Read the model definition and answer for the solid it produces. Units are mm, in the model's axes. Face numbers are marked on the shaded views. A direction names the side the tool comes from. Coordinates: 2 decimals unless noted, no trailing zeros. Loops run counter-clockwise (first coordinate to the right, second up) from the corner with the lowest first, then second, coordinate; pieces in that order, holes last.
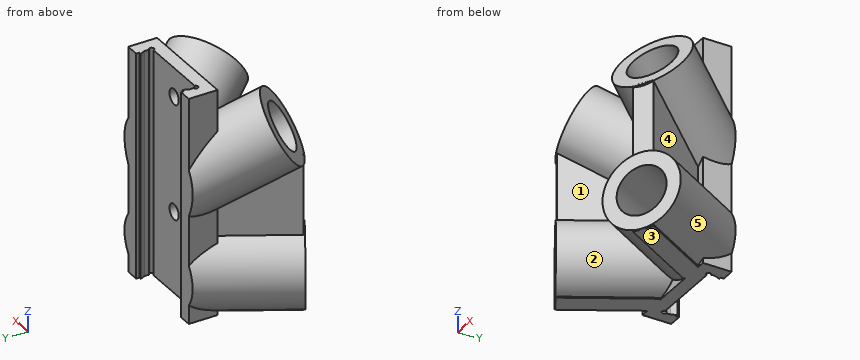
from build123d import *

# Parameters (mm, degrees)
BOSS_EXTRUDE1_DEPTH      = 25
BOSS_EXTRUDE1_DEPTH_BACK = 22
SKETCH5_R                = 8
BOSS_EXTRUDE2_DEPTH      = 30
SKETCH6_R                = 8
BOSS_EXTRUDE3_DEPTH      = 30
SKETCH18_R               = 8
BOSS_EXTRUDE4_DEPTH      = 30
SKETCH19_R               = 8
BOSS_EXTRUDE5_DEPTH      = 30
SKETCH11_R               = 0.5
CUT_EXTRUDE4_DEPTH       = 61.172763276
CUT_EXTRUDE5_REACH       = 41.594
SKETCH12_R               = 1.6
TOPCUT_DEPTH             = 61.172763276
GRABTABS_DEPTH           = 47
BOSS_EXTRUDE6_DEPTH      = 30.5
SKETCH22_R               = 5.1
CUT_EXTRUDE6_DEPTH       = 14
SKETCH23_R               = 5.1
CUT_EXTRUDE7_DEPTH       = 14
SKETCH20_R               = 5.1
CUT_EXTRUDE8_DEPTH       = 14
SKETCH21_R               = 5.1
CUT_EXTRUDE9_DEPTH       = 14


with BuildPart() as part:
    # Sketch3 → Boss-Extrude1 (new, two sides: drawn at the far end of the back side and taken through both)
    with BuildSketch(Plane(origin=(0, 0, 0), x_dir=(-0.9678879191476432, 0.2513821313618881, 0), z_dir=(0, 0, 1)).offset(-BOSS_EXTRUDE1_DEPTH_BACK)):
        Polygon((-7.234103595, -12.967950693), (12.967950693, -7.234103595), (7.234103595, 12.967950693), (-12.967950693, 7.234103595), align=None)
    extrude(amount=BOSS_EXTRUDE1_DEPTH + BOSS_EXTRUDE1_DEPTH_BACK)

    # Sketch5 → Boss-Extrude2 (add)
    with BuildSketch(Plane(origin=(0, 0, 0), x_dir=(-0.7398893525523432, -0.6222846190478576, -0.2555887299474237), z_dir=(0.4497352826512201, -0.740093355961685, 0.499999999999998))):
        with Locations(Location((0, 0, 0), (0, 0, 224.122685504))):
            Circle(SKETCH5_R)
    extrude(amount=BOSS_EXTRUDE2_DEPTH)

    # Sketch6 → Boss-Extrude3 (add)
    with BuildSketch(Plane(origin=(0, 0, 0), x_dir=(-0.7035639492311271, 0.6172392366079582, 0.3521554970945721), z_dir=(-0.4160720061092844, -0.7595288577349761, 0.499999999999998))):
        with Locations(Location((0, 0, 0), (0, 0, 322.705646398))):
            Circle(SKETCH6_R)
    extrude(amount=BOSS_EXTRUDE3_DEPTH)

    # Sketch18 → Boss-Extrude4 (add)
    with BuildSketch(Plane(origin=(0, 0, -14), x_dir=(-0.8770283809411537, 0.48043856945892555, 0), z_dir=(-0.4804385694589255, -0.8770283809411535, 0))):
        with Locations(Location((0, 0, 0), (0, 0, 61.287925102))):
            Circle(SKETCH18_R)
    extrude(amount=BOSS_EXTRUDE4_DEPTH)

    # Sketch19 → Boss-Extrude5 (add)
    with BuildSketch(Plane(origin=(0, 0, -14), x_dir=(-0.8545861965798597, -0.5193095730055144, 0), z_dir=(0.5193095730055143, -0.8545861965798596, 0))):
        with Locations(Location((0, 0, 0), (0, 0, 48.985500334))):
            Circle(SKETCH19_R)
    extrude(amount=BOSS_EXTRUDE5_DEPTH)

    # Sketch11 → Cut-Extrude4 (cut, through all)
    with BuildSketch(Plane(origin=(0, 0, 25), x_dir=(0.967887919147643, -0.25138213136188803, 0), z_dir=(0, 0, 1))):
        with BuildLine():
            ThreePointArc((-4.766381934, -9.44058657), (-4.766628372, -9.424890171), (-4.767367442, -9.409209245))
            Line((-4.767367442, -9.409209245), (-5.339457415, -9.571582654))
            Line((-5.339457415, -9.571582654), (-5.501830825, -8.999492681))
            ThreePointArc((-5.501830825, -8.999492681), (-5.523554594, -9.869378155), (-4.766381934, -9.44058657))
        make_face()
        with BuildLine():
            Line((-5.339457415, -9.571582654), (-4.767367442, -9.409209245))
            ThreePointArc((-4.767367442, -9.409209245), (-5.022796995, -9.003932957), (-5.501830825, -8.999492681))
            Line((-5.501830825, -8.999492681), (-5.339457415, -9.571582654))
        make_face()
        with BuildLine():
            Line((8.999492681, -5.501830825), (9.571582654, -5.339457415))
            Line((9.571582654, -5.339457415), (9.409209245, -4.767367442))
            ThreePointArc((9.409209245, -4.767367442), (9.003932957, -5.022796995), (8.999492681, -5.501830825))
        make_face()
        with BuildLine():
            Line((9.409209245, -4.767367442), (9.571582654, -5.339457415))
            Line((9.571582654, -5.339457415), (8.999492681, -5.501830825))
            ThreePointArc((8.999492681, -5.501830825), (9.561939475, -5.751431903), (9.94058657, -5.266381934))
            ThreePointArc((9.94058657, -5.266381934), (9.782866673, -4.901903771), (9.409209245, -4.767367442))
        make_face()
        with Locations((-5.266381934, -9.44058657)):
            Circle(SKETCH11_R)
        with Locations((9.44058657, -5.266381934)):
            Circle(SKETCH11_R)
        Polygon((-5.339457415, -9.571582654), (9.571582654, -5.339457415), (5.339457415, 9.571582654), (-9.571582654, 5.339457415), align=None)
    extrude(amount=-CUT_EXTRUDE4_DEPTH, mode=Mode.SUBTRACT)

    # Sketch12 → Cut-Extrude5 (cut, up to next)
    with BuildSketch(Plane(origin=(0.235642936, -10.497355496, 0), x_dir=(0.07428415697149086, 0.0016675187230335104, -0.9972357210832067), z_dir=(-0.02244218436129408, 0.9997481424644377, 0)), mode=Mode.PRIVATE) as cut_extrude5_sk1:
        with Locations(Location((-18.947478701, -1.411754543, 0), (0, 0, 274.261167974))):
            Circle(SKETCH12_R)
    cut_extrude5_tool1 = extrude(cut_extrude5_sk1.sketch, amount=CUT_EXTRUDE5_REACH, mode=Mode.PRIVATE) & part.part
    # Sketch12 → Cut-Extrude5 (cut, up to next)
    with BuildSketch(Plane(origin=(0.235642936, -10.497355496, 0), x_dir=(0.07428415697149086, 0.0016675187230335104, -0.9972357210832067), z_dir=(-0.02244218436129408, 0.9997481424644377, 0)), mode=Mode.PRIVATE) as cut_extrude5_sk2:
        with Locations(Location((5.019164388, 0.373972086, 0), (0, 0, 274.261167974))):
            Circle(SKETCH12_R)
    cut_extrude5_tool2 = extrude(cut_extrude5_sk2.sketch, amount=CUT_EXTRUDE5_REACH, mode=Mode.PRIVATE) & part.part
    add(cut_extrude5_tool1.solids().sort_by_distance((0.235643, -10.497355, 19))[0], mode=Mode.SUBTRACT)
    add(cut_extrude5_tool2.solids().sort_by_distance((0.235643, -10.497355, -5.033077))[0], mode=Mode.SUBTRACT)

    # Sketch14 → TopCut (cut, through all)
    with BuildSketch(Plane.XY.offset(25)):
        Polygon((-31.105779731, -5.199391149), (38.352697692, -3.640198499), (37.988721129, 12.574127466), (-33.745248602, 10.963854933), align=None)
    extrude(amount=-TOPCUT_DEPTH, mode=Mode.SUBTRACT)

    # Sketch17 → GrabTabs (add, through all)
    with BuildSketch(Plane(origin=(0, 0, 25), x_dir=(-1, 0, 0), z_dir=(0, 0, -1))):
        Polygon((7.132596783, -5.31140877), (7.607527123, -6.433816222), (7.632470855, -5.322629862), align=None)
        Polygon((-7.888569085, -6.085962364), (-7.363751282, -4.985997097), (-7.863625354, -4.974776005), align=None)
    extrude(amount=GRABTABS_DEPTH)

    # Sketch24 → Boss-Extrude6 (add)
    with BuildSketch(Plane(origin=(0, 0, -22), x_dir=(-1, 0, 0), z_dir=(0, 0, -1))):
        Polygon((-13.818067506, -26.398167405), (-17.409683037, -24.238344439), (-7.909513608, -8.440310713), (-4.317898077, -10.60013368), align=None)
        Polygon((3.837888164, -10.783213448), (7.522803724, -8.786732873), (16.304497418, -24.9951549), (12.619581859, -26.991635476), align=None)
    extrude(amount=-BOSS_EXTRUDE6_DEPTH)

    # Sketch22 → Cut-Extrude6 (cut)
    with BuildSketch(Plane(origin=(-14.413157084, -26.310851428, 0), x_dir=(0.8770283809411535, -0.48043856945892577, 0), z_dir=(-0.4804385694589257, -0.8770283809411534, 0))):
        with Locations((0, -14)):
            Circle(SKETCH22_R)
    extrude(amount=-CUT_EXTRUDE6_DEPTH, mode=Mode.SUBTRACT)

    # Sketch23 → Cut-Extrude7 (cut)
    with BuildSketch(Plane(origin=(-12.482160183, -22.785865732, 15), x_dir=(0.9093316698170122, -0.34752852674676815, 0.22877901425835656), z_dir=(-0.41607200610928446, -0.7595288577349762, 0.4999999999999979))):
        with Locations(Location((0, 0, 0), (0, 0, 270))):
            Circle(SKETCH23_R)
    extrude(amount=-CUT_EXTRUDE7_DEPTH, mode=Mode.SUBTRACT)

    # Sketch20 → Cut-Extrude8 (cut)
    with BuildSketch(Plane(origin=(13.49205848, -22.202800679, 15), x_dir=(-0.893161897719908, -0.37266042750079065, 0.2517658242023739), z_dir=(0.44973528265122, -0.7400933559616851, 0.49999999999999784))):
        with Locations(Location((0, 0, 0), (0, 0, 90))):
            Circle(SKETCH20_R)
    extrude(amount=-CUT_EXTRUDE8_DEPTH, mode=Mode.SUBTRACT)

    # Sketch21 → Cut-Extrude9 (cut)
    with BuildSketch(Plane(origin=(15.57928719, -25.637585897, 0), x_dir=(0.8545861965798595, 0.5193095730055145, 0), z_dir=(0.5193095730055145, -0.8545861965798595, 0))):
        with Locations((0, -14)):
            Circle(SKETCH21_R)
    extrude(amount=-CUT_EXTRUDE9_DEPTH, mode=Mode.SUBTRACT)


solid = part.part
Q1. Flat-ended cylindrical pins translate along their axes: pin 1 Ø12 at (x, y) = (10, -15.5) entering from +Z; pin 2 Ø4 at (x, z) = (-4, 2.5) entering from +Y; pin 3 Ø1.5 at (x, y) = (-10.5, -26) entering from +Z; pin 4 Ø6 at (x, z) = (-1, 11.5) entering from -Y. Find the tip coordinate at first contact, or state that the pin passes through.
Findings below:
pin 1: stops at z = 25
pin 2: stops at y = -7.8
pin 3: stops at z = 12.24
pin 4: stops at y = -23.76
Q2. Which of the six approach directions +Z, -Z, +X, -X, +Y, -Y give full straight-line access (tool end or side, diameter ignored) to the marked faces 1 and 2?
Findings below:
face 1: -Y
face 2: none
Q3. A cutting plane is placed at C-C (z = -12.5). Give the vertices of the cut face in (x, y).
Findings below:
outline: (-21.3, -22.54) - (-18.69, -23.97) - (-11.96, -11.69) - (-3.41, -16.37) - (-10.14, -28.65) - (-7.52, -30.09) - (0.35, -15.71) - (8.86, -29.72) - (11.41, -28.17) - (4.14, -16.2) - (12.47, -11.14) - (19.74, -23.11) - (22.29, -21.56) - (11.77, -4.24) - (7.85, -4.32) - (7.86, -4.97) - (7.36, -4.99) - (7.89, -6.09) - (7.91, -6.98) arc R0.5 cw (long way) to (7.33, -7.59) - (-6.98, -7.91) arc R0.5 cw (long way) to (-7.59, -7.33) - (-7.61, -6.43) - (-7.13, -5.31) - (-7.63, -5.32) - (-7.65, -4.67) - (-11.57, -4.76) - close
Q4. A cutting plane is placed at A-A (y = -19.75). Count the separate pieces of the cut face and the enclosed holes in it, then the cut area to 3 significant figures.
Findings below:
separate pieces: 2
enclosed holes: 2
area: 605 mm2
Q5. Determine the mould class of the marked faces 3, 4 and 5 for opening direction X: +X half, -X half, draft (parallel to the pull), parting line (faces both ways), or undercut.
Findings below:
face 3: draft
face 4: +X half
face 5: undercut
Q6. Straight lines are drawn through the part: probe 1 along X at (y, z) = (-14.5, 13); probe 2 along X at (y, z) = (-12.5, 5); probe 3 along Z at (x, y) = (-8, -15). For each, find the intervals that lie inside material, in ascending order.
Findings below:
probe 1: x = -17.02 to -13.44, -4.19 to -0.61, 1.27 to 4.84, 14.59 to 18.16
probe 2: x = -14.32 to -10.8, -9.63 to 9.45, 11.36 to 14.99
probe 3: z = -22 to -19.1, -8.9 to 3.93, 15.7 to 19.05
